from build123d import *

# Parameters (mm, degrees)
SKETCH_1_W          = 60
SKETCH_1_H          = 30
EXTRUDE_1_DEPTH     = 3
SKETCH_2_W          = 3
SKETCH_2_H          = 30
EXTRUDE_2_DEPTH     = 6
SKETCH_3_R          = 10.5
CUT_EXTRUDE_1_DEPTH = 6
FILLET_1_R          = 10
SKETCH_4_W          = 26.464102696
SKETCH_4_H          = 3.3
CUT_EXTRUDE_2_DEPTH = 6


with BuildPart() as part:
    # 草图1 → 凸台-拉伸1 (new body)
    with BuildSketch(Plane.XY):
        with Locations((30, 15)):
            Rectangle(SKETCH_1_W, SKETCH_1_H)
    extrude(amount=EXTRUDE_1_DEPTH)

    # 草图2 → 凸台-拉伸2 (add)
    with BuildSketch(Plane.XY.offset(3)):
        with Locations((1.5, 15)):
            Rectangle(SKETCH_2_W, SKETCH_2_H)
    extrude(amount=EXTRUDE_2_DEPTH)

    # 草图3 → 切除-拉伸1 (cut)
    with BuildSketch(Plane.XY.offset(3)):
        with Locations((47, 15)):
            Circle(SKETCH_3_R)
    extrude(amount=-CUT_EXTRUDE_1_DEPTH, mode=Mode.SUBTRACT)

    # 圆角1
    fillet_1_edges = [part.edges().sort_by_distance(p)[0] for p in [
        (60, 30, 1.5),
        (60, 0, 1.5),
    ]]
    fillet(fillet_1_edges, radius=FILLET_1_R)

    # 草图4 → 切除-拉伸2 (cut)
    with BuildSketch(Plane.XY.offset(3)):
        with Locations((18.373081002, 15)):
            Rectangle(SKETCH_4_W, SKETCH_4_H)
    extrude(amount=-CUT_EXTRUDE_2_DEPTH, mode=Mode.SUBTRACT)


solid = part.part
Verification items for the finished model (mm, model axes). A direction names the side the tool comes from. Coordinates: 2 decimals unless noted, no trailing zeros. Write each loop counter-clockwise with the first axis right and the second up, starting at its lowest first coordinate (ties: lowest second). Pieces come first, ordered by that corner, then holes. Notation, with made-up numbers: M -25.75,47 L 16.25,47 A28 ccw 16.25,79 Z; hole C -33.5,1 d1. An arc over 180 degrees is marked long. Use CSV: the item, a comma, the result in double quotes.
Q1. Section check B-B, the plane y = 15. Enter the section's corners in (x, z).
Computed values:
outline,"M 0,0 L 5.14,0 L 5.14,3 L 3,3 L 3,9 L 0,9 Z; M 31.61,0 L 36.5,0 L 36.5,3 L 31.61,3 Z; M 57.5,0 L 60,0 L 60,3 L 57.5,3 Z"
Q2. Set-up check for faces 1 (the flat face through (18, 13.35, 2)), 2 (the flat face through (19, 30, 2)), 3 (the flat face through (25, 19, 3)): record each of +Z, -Z, +X, -X, +Y, -Y from which the full face is reachable in a straight line by a thin tool's end or side.
Computed values:
face 1,"+Z, -Z"
face 2,"+Z, -Z, +X, -X, +Y"
face 3,"+Z, +X, +Y, -Y"
Q3. Section check D-D, the plane y = 23.75. Enter the section's corners in (x, z).
Computed values:
outline,"M 0,0 L 41.2,0 L 41.2,3 L 3,3 L 3,9 L 0,9 Z; M 52.8,0 L 59.27,0 L 59.27,3 L 52.8,3 Z"
Q4. Section check C-C, the plane x = 47. Enter the section's corners in (y, z), and give its area (3 significant figures).
Computed values:
outline,"M 0,0 L 4.5,0 L 4.5,3 L 0,3 Z; M 25.5,0 L 30,0 L 30,3 L 25.5,3 Z"
area,"27.0 mm²"
Q5. Section check A-A, the plane z = 2.25. Enter the section's corners in (x, y).
Computed values:
outline,"M 0,0 L 50,0 A10 ccw 60,10 L 60,20 A10 ccw 50,30 L 0,30 Z; hole M 5.14,13.35 L 31.61,13.35 L 31.61,16.65 L 5.14,16.65 Z; hole C 47,15 d21"
Q6. Mould release check, pull along X, two halves, no side actions. Record for faces 4 (the flat face through (1, 15, 9)), 5 (the cylindrical face through (56.99, 27.15, 1.52)), 6 (the flat face through (18, 16.65, 2)): pulls with the +X half, pulls with the -X half, needs draft (parallel to the pull), parting line crosses it, or undercut.
Computed values:
face 4,"needs draft"
face 5,"pulls with the +X half"
face 6,"undercut"
Q7. Go/stop test with flat-tipped pins: P1, Ø3, axis at x = 17, y = 9, coming from the +Z side; P2, Ø1.8, axis at y = 18.5, z = 4.5, coming from the +X side; P3, Ø12, axis at x = 44, y = 15, coming from the +Z side. Record where each tip stops, or that it passes through.
Computed values:
P1,"z = 3"
P2,"x = 3"
P3,"through"
Q8. Thickness scan on line 1 along Y through (x, z) = (47, 1.15); line 2 along Y through (x, z) = (12, 2); line 3 along Z through (x, y) = (6.5, 6.25). Record the ranges inside material, lowest first. Write a range as [from, to].
Computed values:
line 1,"[0, 4.5], [25.5, 30]"
line 2,"[0, 13.35], [16.65, 30]"
line 3,"[0, 3]"
